Design review of the part built by this model. Coordinates are the model's own, in mm. Face numbers are marked on the shaded views. A direction names the side the tool comes from. Coordinates: 2 decimals unless noted, no trailing zeros. Loops run counter-clockwise (first coordinate to the right, second up) from the corner with the lowest first, then second, coordinate; pieces in that order, holes last. Notation, with made-up numbers: M 89,75.5 L 110,75.5 A22 ccw 110,81.5 Z; hole C 48.5,24 d4. An arc over 180 degrees is marked long. One line per item, written item: value.
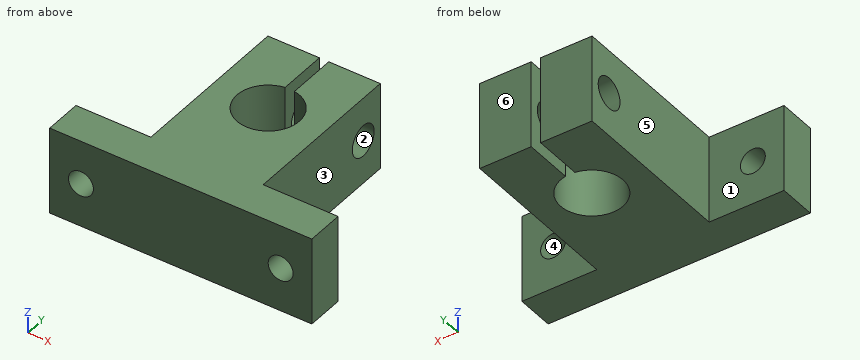
```python
from build123d import *

# Parameters (mm, degrees)
BOSS_EXTRUDE1_DEPTH = 14
SKETCH2_R           = 2.5
CUT_EXTRUDE1_DEPTH  = 37.945365068
SKETCH3_R           = 2
CUT_EXTRUDE2_DEPTH  = 14


with BuildPart() as part:
    # Sketch1 → Boss-Extrude1 (new body)
    with BuildSketch(Plane.XY):
        with BuildLine():
            Line((-21, -16.4), (21, -16.4))
            Line((21, -16.4), (21, -10.4))
            Line((21, -10.4), (9, -10.4))
            Line((9, -10.4), (9, 16.4))
            Line((9, 16.4), (0.75, 16.4))
            Line((0.75, 16.4), (0.75, 8.543429983))
            ThreePointArc((0.75, 8.543429983), (0, -1.4), (-0.75, 8.543429983))
            Line((-0.75, 8.543429983), (-0.75, 16.4))
            Line((-0.75, 16.4), (-9, 16.4))
            Line((-9, 16.4), (-9, -10.4))
            Line((-9, -10.4), (-21, -10.4))
            Line((-21, -10.4), (-21, -16.4))
        make_face()
    extrude(amount=BOSS_EXTRUDE1_DEPTH)

    # Sketch2 → Cut-Extrude1 (cut, through all)
    with BuildSketch(Plane(origin=(9, 0, 0), x_dir=(0, 0, -1), z_dir=(1, 0, 0))):
        with Locations((-7, 12.5)):
            Circle(SKETCH2_R)
    extrude(amount=-CUT_EXTRUDE1_DEPTH, mode=Mode.SUBTRACT)

    # Sketch3 → Cut-Extrude2 (cut)
    with BuildSketch(Plane(origin=(0, -10.4, 0), x_dir=(1, 0, 0), z_dir=(0, 1, 0))):
        with Locations(Location((-16, -7, 0), (0, 0, 180))):
            Circle(SKETCH3_R)
        with Locations(Location((16, -7, 0), (0, 0, 180))):
            Circle(SKETCH3_R)
    extrude(amount=-CUT_EXTRUDE2_DEPTH, mode=Mode.SUBTRACT)


solid = part.part
```
(1) To check wall thickness, follow line 1 along Z through (x, y) = (16, -12); line 2 along X through (y, z) = (13, 9.75). State the ranges of each line that lie inside material, in increasing order. Write a range as [from, to].
Reply:
line 1: z = [0, 5], [9, 14]
line 2: x = [-9, -0.75], [0.75, 9]
(2) Tool access review of the marked faces 1, 2 and 3: name each direction out of +Z, -Z, +X, -X, +Y, -Y from which nothing blocks a thin tool from reaching the whole face with its end or side.
Reply:
face 1: +Z, -Z, -X, +Y
face 2: +X, -X
face 3: +Z, -Z, +X, +Y
(3) We need section D-D on x = -2.5. State the section outline as (y, z) points, then the cut area to 3 significant figures.
Reply:
outline: M -16.4,0 L -0.73,0 L -0.73,14 L -16.4,14 Z; M 7.93,0 L 16.4,0 L 16.4,14 L 7.93,14 Z; hole C 12.5,7 d5
area: 318 mm2
(4) We need section A-A on z = 7. State the section outline as (x, y) points, then the cut area to 3 significant figures.
Reply:
outline: M -21,-16.4 L -18,-16.4 L -18,-10.4 L -21,-10.4 Z; M -14,-16.4 L 14,-16.4 L 14,-10.4 L 9,-10.4 L 9,10 L 0.75,10 L 0.75,8.54 A5 cw long -0.75,8.54 L -0.75,10 L -9,10 L -9,-10.4 L -14,-10.4 Z; M -9,15 L -0.75,15 L -0.75,16.4 L -9,16.4 Z; M 0.75,15 L 9,15 L 9,16.4 L 0.75,16.4 Z; M 18,-16.4 L 21,-16.4 L 21,-10.4 L 18,-10.4 Z
area: 514 mm2
(5) We need section C-C on x = 16. State the section outline as (y, z) points, then the cut area to 3 significant figures.
Reply:
outline: M -16.4,0 L -10.4,0 L -10.4,5 L -16.4,5 Z; M -16.4,9 L -10.4,9 L -10.4,14 L -16.4,14 Z
area: 60.0 mm2
(6) Mouldability with a two-part tool opening along X and no side actions: class the marked faces 4, 5 and 6 as released by +X, released by -X, zero draft, split by the parting line, or undercut.
Reply:
face 4: undercut
face 5: released by -X
face 6: zero draft
(7) We need section B-B on y = 11. State the section outline as (x, z) points.
Reply:
outline: M -9,0 L -0.75,0 L -0.75,5 L -9,5 Z; M -9,9 L -0.75,9 L -0.75,14 L -9,14 Z; M 0.75,0 L 9,0 L 9,5 L 0.75,5 Z; M 0.75,9 L 9,9 L 9,14 L 0.75,14 Z
(8) Insertion check: pin 1 (1.5 mm diameter, centred on y = -3, z = 3.5, fed in from +X); pin 2 (6.5 mm diameter, centred on y = 14.5, z = 10, fed in from -X); pin 3 (8 mm diameter, centred on x = -3.5, y = 11, fed in from -Z); pin 4 (6 mm diameter, centred on x = -12.5, z = 10, fed in from +Y). Each pin has a flat end and moves straight along its axis. Give the tip position at first contact, or say it passes through.
Reply:
pin 1: stops at x = 9
pin 2: stops at x = -9
pin 3: stops at z = 0
pin 4: stops at y = -10.4
